Job drawing, mm, ordinate dimensions from the low corner. One solid piece. A direction names the side the tool comes from. Give positions to 0.01 mm unless a question says otherwise; leave off trailing zeros. Write each loop counter-clockwise with the first axis right and the second up, starting at its lowest first coordinate (ties: lowest second). Pieces come first, ordered by that corner, then holes. Notation, with made-up numbers: (40.25, -9) - (56.25, -9) arc R17 cw to (56.25, 12) - close; hole circle Ø9 at (51, 84). An arc over 180 degrees is marked (long way). Answer in a Markdown table with one row per item. Add a question column.
1. Band-saw the part on B-B on z = 73. Write the cut outline in (x, y).
2. Drop flat-ended pins along their axis: pin 1 Ø3.5 at (x, y) = (45, 2) entering from -Z; pin 2 Ø1.5 at (x, y) = (44, 1) entering from -Z; pin 3 Ø3.5 at (x, y) = (19, 1) entering from +Z. Give the stop position or say it passes through.
3. Band-saw the part on C-C on y = 37.5. Write the cut outline in (x, z), plus the area to 3 significant figures.
4. Probe line 1 along Z through (x, y) = (36, 117.5); line 2 along Y through (x, z) = (49.5, 69.5); line 3 along Y through (x, z) = (39, 5). List the from-to ranges inside material, lowest first.
5. Band-saw the part on D-D on x = 55.5. Write the cut outline in (y, z), plus the area to 3 significant figures.
6. Band-saw the part on A-A on x = 43.5. Write the cut outline in (y, z).
7. Which spindle directions (+Z, -Z, +X, -X, +Y, -Y) get a long thin tool onto all of the face, cutting with end or side? Do the marked faces 1 and 2. Say none if no direction does.
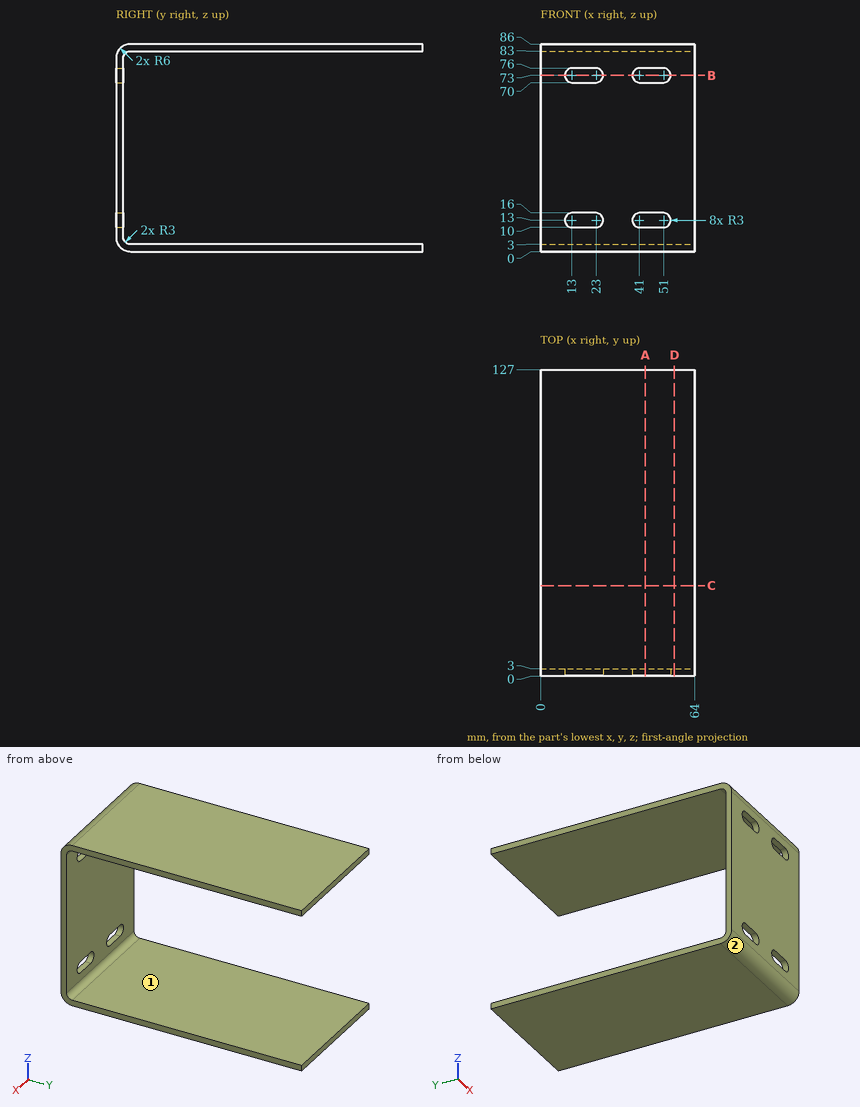
Values:
| question | item | result |
|---|---|---|
| 1 | outline | (0, 0) - (10, 0) - (10, 3) - (0, 3) - close; (26, 0) - (38, 0) - (38, 3) - (26, 3) - close; (54, 0) - (64, 0) - (64, 3) - (54, 3) - close |
| 2 | pin 1 | stops at z = 0.44 |
| 2 | pin 2 | stops at z = 1.76 |
| 2 | pin 3 | stops at z = 85.04 |
| 3 | outline | (0, 0) - (64, 0) - (64, 3) - (0, 3) - close; (0, 83) - (64, 83) - (64, 86) - (0, 86) - close |
| 3 | area | 384 mm² |
| 4 | line 1 | z = 0 to 3, 83 to 86 |
| 4 | line 2 | y = 0 to 3 |
| 4 | line 3 | y = 0.08 to 3.17 |
| 5 | outline | (0, 6) arc R6 ccw to (6, 0) - (127, 0) - (127, 3) - (6, 3) arc R3 cw to (3, 6) - (3, 80) arc R3 cw to (6, 83) - (127, 83) - (127, 86) - (6, 86) arc R6 ccw to (0, 80) - close |
| 5 | area | 990 mm² |
| 6 | outline | (0, 6) arc R6 ccw to (6, 0) - (127, 0) - (127, 3) - (6, 3) arc R3 cw to (3, 6) - (3, 10) - (0, 10) - close; (0, 16) - (3, 16) - (3, 70) - (0, 70) - close; (0, 76) - (3, 76) - (3, 80) arc R3 cw to (6, 83) - (127, 83) - (127, 86) - (6, 86) arc R6 ccw to (0, 80) - close |
| 7 | face 1 | +X, -X, +Y |
| 7 | face 2 | -Z, +X, -X, -Y |
